For this review, take the finished solid that the model builds, in its own axes (mm). A direction names the side the tool comes from. Coordinates: 2 decimals unless noted, no trailing zeros. Loops run counter-clockwise (first coordinate to the right, second up) from the corner with the lowest first, then second, coordinate; pieces in that order, holes last.
1. Take a section at A-A, the plane y = 0. State the section outline as (x, z) points, then the cut area to 3 significant figures.
2. Machinability: for faces 4 (the face through (-2.3, -2.3, 0)), 5 (the face through (2, -10, 18)), 6 (the face through (-0.07, -5.51, 10.89)), which of the approach directions +Z, -Z, +X, -X, +Y, -Y give a long, thin tool a straight path to every point of the face, cutting with its end or side? Answer none if there is none.
3. Take a section at B-B, the plane x = 0. State the section outline as (y, z) points.
4. Take a section at C-C, the plane z = 14.25. State the section outline as (x, y) points.
5. To check wall thickness, follow probe 1 along Y at (x, z) = (0, 5.5); probe 2 along Z at (x, y) = (0, -6.1); probe 3 along Z at (x, y) = (8, 6.5). State the ranges of each line that lie inside material, in increasing order.
6. Mouldability with a two-part tool opening along X and no side actions: class faces 1 (the face through (-2, -10, 2)), 2 (the face through (-2.38, -10.74, 19.01)), 3 (the face through (0, 3, 10)) as pulls with the +X half, pulls with the -X half, needs draft (parallel to the pull), parting line crosses it, or undercut.
7. Clearance check with flat-ended pins moving along their axes: P1, Ø4, axis at x = 0, z = 9.39, coming from the +Y side; P2, Ø5, axis at x = -7.5, y = -8.5, coming from the +Z side; P3, Ø1.5, axis at y = -8.5, z = 16, coming from the -X side; P4, Ø5, axis at x = 4, z = 6, coming from the +Y side. State where each tip first meets the part, or that it passes through.
8. Take a section at D-D, the plane y = -5.5. State the section outline as (x, z) points.
Autodesk Inventor part; units mm, degrees
ref_plane "YZ Plane" through (0, 0, 0) normal (1, 0, 0) x (0, 1, 0)
ref_plane "XZ Plane" through (0, 0, 0) normal (0, 1, 0) x (-1, 0, 0)
ref_plane "XY Plane" through (0, 0, 0) normal (0, 0, 1) x (1, 0, 0)
sketch "Sketch1" plane through (0, 0, 0) normal (0, 0, 1) x (1, 0, 0)
  circle A0 centre (0, 0) radius 10
  dimension "d0" = 20
extrude "Extrusion1" add sketch "Sketch1" along normal blind 20
sketch "Sketch2" plane through (0, 0, 20) normal (0, 0, 1) x (1, 0, 0)
  circle A0 centre (0, 0) radius 11
  dimension "d3" = 22
extrude "Extrusion2" add sketch "Sketch2" against normal blind 2
sketch "Sketch3" plane through (0, 0, 0) normal (0, 0, -1) x (-1, 0, 0)
  circle A0 centre (0, 0) radius 11
extrude "Extrusion3" add sketch "Sketch3" against normal blind 2
sketch "Sketch4" plane through (0, 0, 0) normal (0, 1, 0) x (-1, 0, 0)
  circle A0 centre (0, 9.3897) radius 1.5
  point P0 (0, 0)
  dimension "d8" = 3
extrude "Extrusion4" add sketch "Sketch4" against normal blind 10
sketch "Sketch5" plane through (0, -10, 0) normal (0, -1, 0) x (1, 0, 0)
  arc A0 (0, 7.8897) -> (0, 10.8897) centre (0, 9.3897) ccw
  point P0 (0, 0)
hole "Hole1" at (0, -10, 9.3897) direction (0, 1, 0) diameter 3 depth 10 tip angle 118 countersink diameter 6 countersink angle 90
sketch "Sketch6" plane through (0, 0, 0) normal (0, 0, -1) x (-1, 0, 0)
  circle A0 centre (0, 0) radius 3
  dimension "d18" = 6
extrude "Extrusion5" cut sketch "Sketch6" against normal blind 20
properties part number "bearing v3"
Results list:
1. outline: (-11, 0) - (-3, 0) - (-3, 20) - (-11, 20) - (-11, 18) - (-10, 18) - (-10, 2) - (-11, 2) - close; (3, 0) - (11, 0) - (11, 2) - (10, 2) - (10, 18) - (11, 18) - (11, 20) - (3, 20) - close
1. area: 288 mm2
2. face 4: -Z, +X, -X, +Y, -Y
2. face 5: none
2. face 6: -Y
3. outline: (-11, 0) - (-3, 0) - (-3, 7.89) - (-8.5, 7.89) - (-10, 6.39) - (-10, 2) - (-11, 2) - close; (-11, 18) - (-10, 18) - (-10, 12.39) - (-8.5, 10.89) - (-3, 10.89) - (-3, 20) - (-11, 20) - close; (3, 0) - (11, 0) - (11, 2) - (10, 2) - (10, 18) - (11, 18) - (11, 20) - (3, 20) - close
4. outline: circle Ø20 at (0, 0); hole circle Ø6 at (0, 0)
5. probe 1: y = -10 to -3, 3 to 10
5. probe 2: z = 0 to 7.89, 10.89 to 20
5. probe 3: z = 0 to 2, 18 to 20
6. face 1: needs draft
6. face 2: parting line crosses it
6. face 3: undercut
7. P1: stops at y = 10
7. P2: stops at z = 20
7. P3: stops at x = -6.32
7. P4: stops at y = 9.89
8. outline: (-9.53, 0) - (9.53, 0) - (9.53, 2) - (8.35, 2) - (8.35, 18) - (9.53, 18) - (9.53, 20) - (-9.53, 20) - (-9.53, 18) - (-8.35, 18) - (-8.35, 2) - (-9.53, 2) - close; hole circle Ø3 at (0, 9.39)
